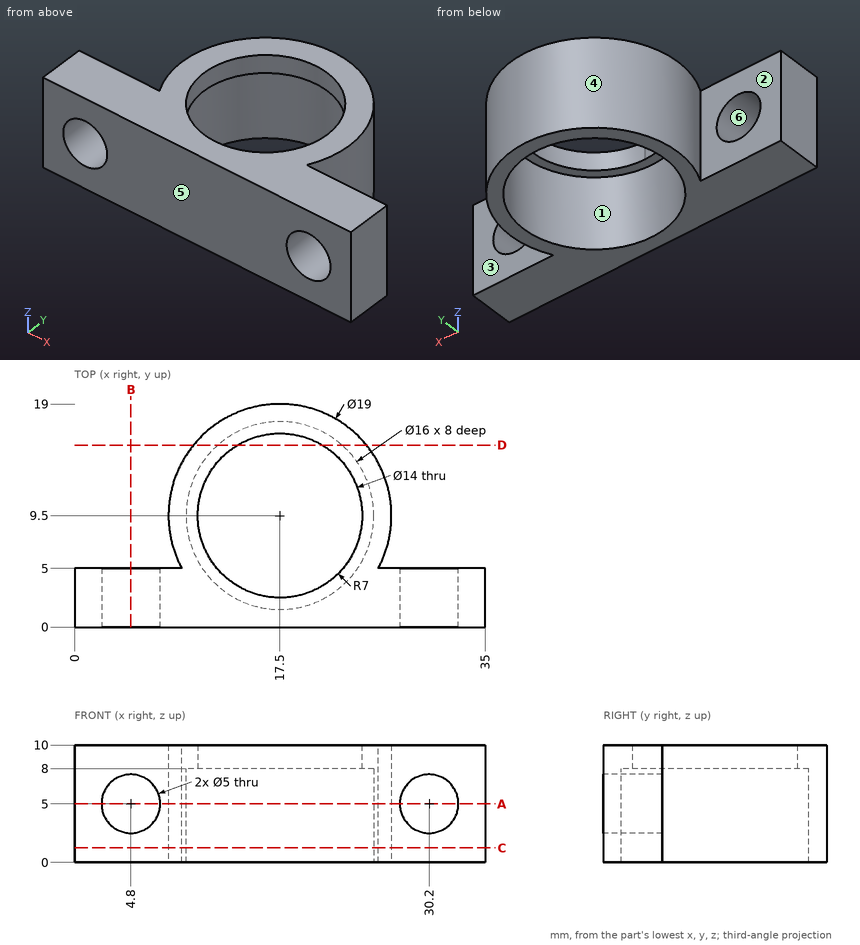
Geometry: see drawing. Coordinates: mm, zero at the bounding-box minimum. A direction names the side the tool comes from. Round coordinates to 2 decimals unless told otherwise and drop trailing zeros. Order: outer loops, then holes, each group sorted by start corner. A loop starts at its lowest first (then second) coordinate and runs counter-clockwise, first axis right, second up. Notation, with made-up numbers: (12, 10) -> (43, 10) arc R20 ccw to (43, 38) -> close; hole circle Ø7 at (45, 53.5). An arc over 180 degrees is marked (long way). Use CSV: the item, a comma, the result in double quotes.
(1) Section D-D on y = 15.5. Return the cut outline in (x, z), and give its area (3 significant figures).
Report:
outline,"(10.13, 0) -> (12.21, 0) -> (12.21, 8) -> (13.89, 8) -> (13.89, 10) -> (10.13, 10) -> close; (21.11, 8) -> (22.79, 8) -> (22.79, 0) -> (24.87, 0) -> (24.87, 10) -> (21.11, 10) -> close"
area,"48.2 mm^2"
(2) Ray query, L1, parallel to Z at x = 30.2, y = 1.55; L2, parallel to X at y = 2.25, z = 5.5; L3, parallel to Y at x = 7, z = 8.75. Return the intervals inside material, ascending.
Report:
L1,"0 to 2.5, 7.5 to 10"
L2,"0 to 2.35, 7.25 to 14.12, 20.88 to 27.75, 32.65 to 35"
L3,"0 to 5"
(3) Section C-C on z = 1.25. Return the cut outline in (x, y).
Report:
outline,"(0, 0) -> (35, 0) -> (35, 5) -> (25.87, 5) arc R9.5 ccw (long way) to (9.13, 5) -> (0, 5) -> close; hole circle Ø16 at (17.5, 9.5)"
(4) Section B-B on x = 4.8. Return the cut outline in (y, z).
Report:
outline,"(0, 0) -> (5, 0) -> (5, 2.5) -> (0, 2.5) -> close; (0, 7.5) -> (5, 7.5) -> (5, 10) -> (0, 10) -> close"
(5) Pull-direction query (Y, two-part tool) for the marked faces 4, 5 and 6; classes: +Y half, -Y half, draft (parallel to the pull), parting line (faces both ways), or undercut.
Report:
face 4,"undercut"
face 5,"-Y half"
face 6,"draft"
(6) Access query for the marked faces 1, 2 and 3. Directions: +Z, -Z, +X, -X, +Y, -Y. A direction counts if a zero-diameter tool reaches every point of the face in a straight line with its end or side. Return the directions, or none.
Report:
face 1,"-Z"
face 2,"+Z, -Z, -X"
face 3,"+Z, -Z, +X"
(7) First-contact query: pin 1 Ø2.5 at (x, z) = (3, 3) entering from +Y; pin 2 Ø5 at (x, z) = (23.5, 5.5) entering from +Y; pin 3 Ø3 at (y, z) = (8, 8) entering from -X; pin 4 Ø11 at (x, y) = (17.5, 9.5) entering from +Z. Flat tips, straight axial feed; report the tip coordinate or a pass-through.
Report:
pin 1,"y = 5"
pin 2,"y = 18.33"
pin 3,"x = 8"
pin 4,"through"
(8) Section A-A on z = 5. Return the cut outline in (x, y).
Report:
outline,"(0, 0) -> (2.3, 0) -> (2.3, 5) -> (0, 5) -> close; (7.3, 0) -> (27.7, 0) -> (27.7, 5) -> (25.87, 5) arc R9.5 ccw (long way) to (9.13, 5) -> (7.3, 5) -> close; (32.7, 0) -> (35, 0) -> (35, 5) -> (32.7, 5) -> close; hole circle Ø16 at (17.5, 9.5)"
